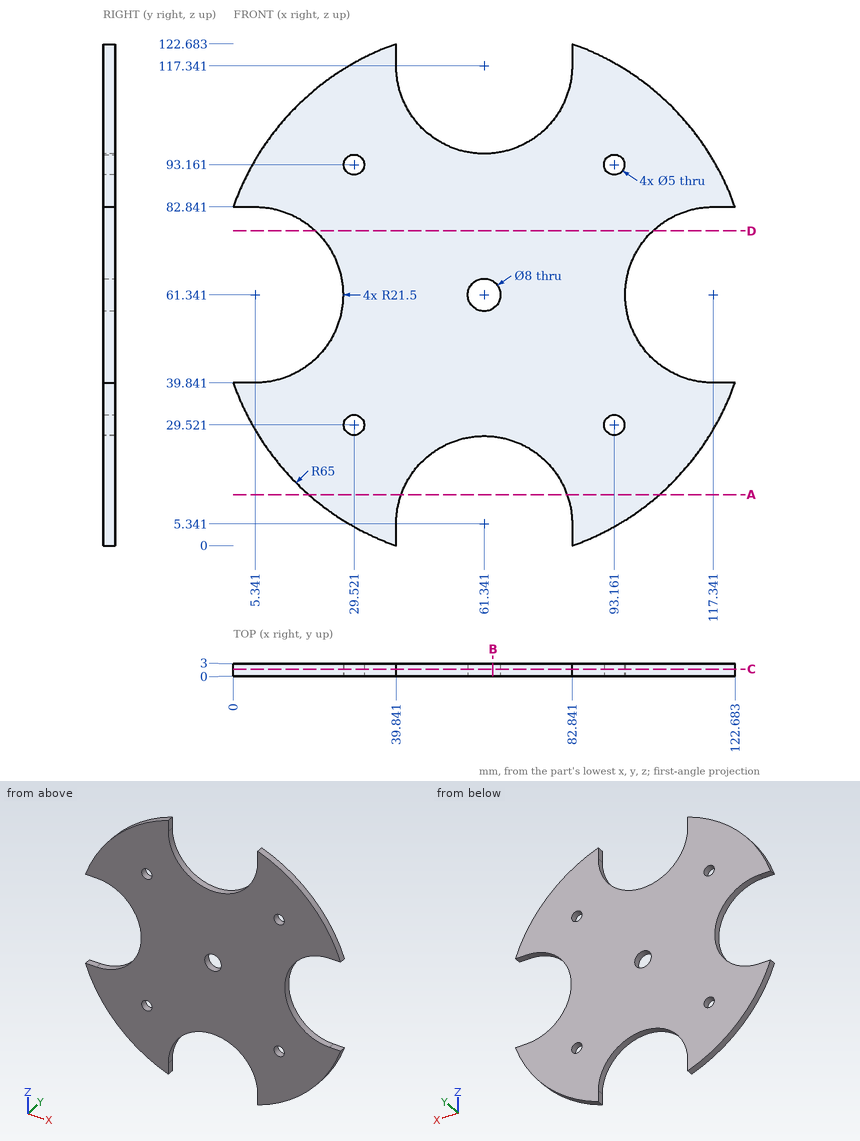
The figure shows three views and two pictorial views of one solid part (mm, origin at its lowest corner). Answer the questions. Coordinates: 2 decimals unless noted, no trailing zeros. Loops run counter-clockwise (first coordinate to the right, second up) from the corner with the lowest first, then second, coordinate; pieces in that order, holes last. Notation, with made-up numbers: (4.25, -5.75) - (55.25, -5.75) arc R29 cw to (55.25, 25.25) - close; hole circle Ø1 at (-6, 70). An arc over 180 degrees is marked (long way). Answer in a Markdown table with one row per item.
Q1. Find section B-B on x = 63.5. Write down the section's boundary in (y, z).
Here are the results:
| item | result |
|---|---|
| outline | (0, 26.73) - (3, 26.73) - (3, 57.97) - (0, 57.97) - close; (0, 64.71) - (3, 64.71) - (3, 95.95) - (0, 95.95) - close |
Q2. Find section D-D on z = 77. Write down the section's boundary in (x, y).
Here are the results:
| item | result |
|---|---|
| outline | (20.07, 0) - (102.61, 0) - (102.61, 3) - (20.07, 3) - close |
Q3. Given P1, Ø1.5, axis at y = 1.5, z = 119.5, coming from the -X side (1 decimal); P2, Ø0.9, axis at y = 1, z = 3, coming from the +X side (1 decimal), each flat-ended and moving along its own axis, determine where each tip first touches the part or whether it passes through.
Here are the results:
| item | result |
|---|---|
| P1 | stops at x = 30.9 |
| P2 | stops at x = 90.9 |
Q4. Find section C-C on y = 1.65. Write down the section's boundary in (x, z), plus the area to 3 significant figures.
Here are the results:
| item | result |
|---|---|
| outline | (0, 39.84) arc R65 ccw to (39.84, 0) - (39.84, 5.34) arc R21.5 cw to (82.84, 5.34) - (82.84, 0) arc R65 ccw to (122.68, 39.84) - (117.34, 39.84) arc R21.5 cw to (117.34, 82.84) - (122.68, 82.84) arc R65 ccw to (82.84, 122.68) - (82.84, 117.34) arc R21.5 cw to (39.84, 117.34) - (39.84, 122.68) arc R65 ccw to (0, 82.84) - (5.34, 82.84) arc R21.5 cw to (5.34, 39.84) - close; hole circle Ø5 at (29.52, 29.52); hole circle Ø5 at (29.52, 93.16); hole circle Ø8 at (61.34, 61.34); hole circle Ø5 at (93.16, 29.52); hole circle Ø5 at (93.16, 93.16) |
| area | 8,900 mm^2 |
Q5. Find section A-A on z = 12.5. Write down the section's boundary in (x, y) (1 decimal), plus the area to 3 significant figures.
Here are the results:
| item | result |
|---|---|
| outline | (18.5, 0) - (41.1, 0) - (41.1, 3) - (18.5, 3) - close; (81.6, 0) - (104.2, 0) - (104.2, 3) - (81.6, 3) - close |
| area | 136 mm^2 |
Q6. Straight lines are drawn through the part: line 1 along Z through (x, y) = (91.5, 1.4) (1 decimal); line 2 along X through (y, z) = (2.9, 94) (1 decimal); line 3 along Z through (x, y) = (64, 2.25) (1 decimal). For each, find the intervals that lie inside material, in ascending order. Write a range as [from, to].
Here are the results:
| item | result |
|---|---|
| line 1 | z = [3.8, 27.7], [31.4, 91.3], [95, 118.9] |
| line 2 | x = [5.1, 27.2], [31.9, 90.8], [95.5, 117.5] |
| line 3 | z = [26.7, 58.4], [64.3, 96] |
